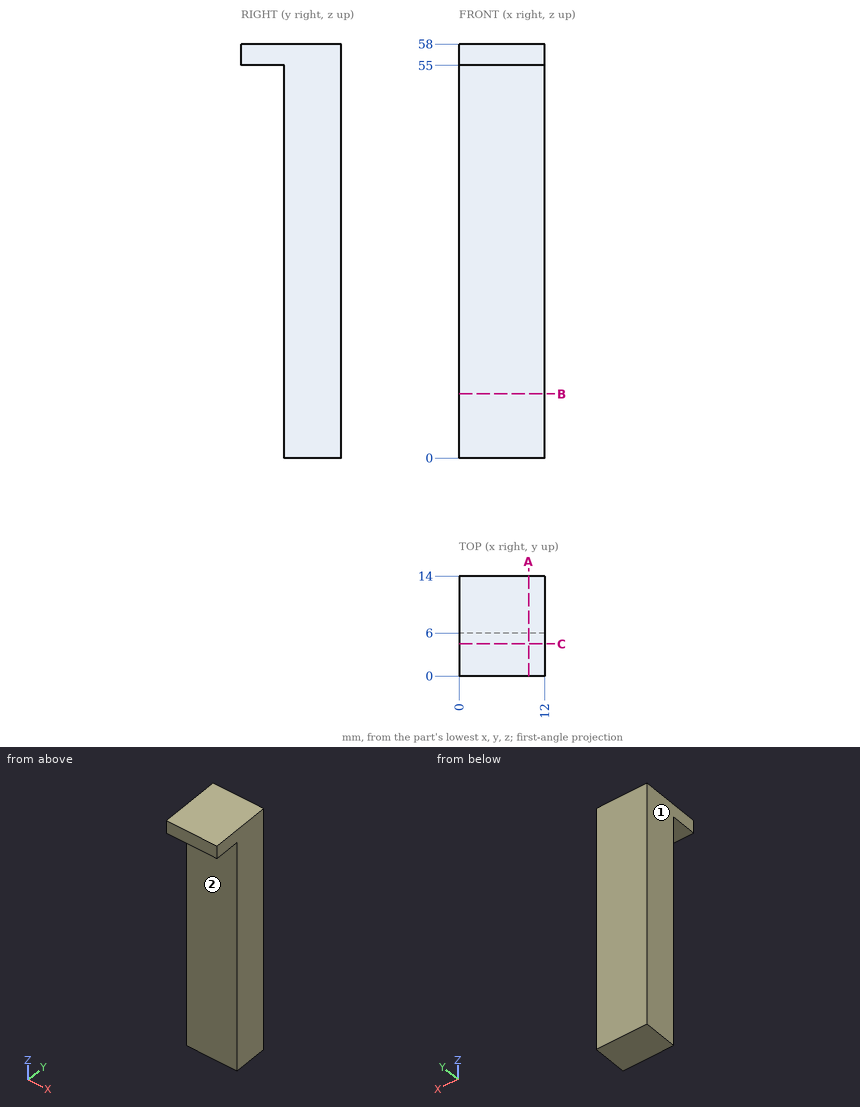
Job drawing, mm, ordinate dimensions from the low corner. One solid piece. A direction names the side the tool comes from. Coordinates: 2 decimals unless noted, no trailing zeros. Order: outer loops, then holes, each group sorted by start corner. A loop starts at its lowest first (then second) coordinate and runs counter-clockwise, first axis right, second up. Notation, with made-up numbers: (14.5, 30) -> (29.5, 30) arc R21 cw to (29.5, 68) -> close; hole circle Ø8 at (0.25, -28.5). An arc over 180 degrees is marked (long way). Return JSON: item names as keys, results as strings. Group by question number.
Item 1: Saw through at C-C on y = 4.5. Write the cut outline in (x, z), then the cut area to 3 significant figures.
Item 2: Flat gauge pins, fed straight in: P1, Ø3, axis at x = 5.5, z = 37, coming from the -Y side; P2, Ø1.8, axis at x = 4, y = 3, coming from the -Z side. Where does each tip first touch, or does it go through?
Item 3: Wall check: line 1 along Y through (x, z) = (10.5, 9); line 2 along Z through (x, y) = (7, 4.5). Give the ranges that are in metal, low to high. Write a range as [from, to].
Item 4: Saw through at A-A on x = 9.75. Write the cut outline in (y, z).
Item 5: Tool access for the marked faces 1 and 2: list every direction of +Z, -Z, +X, -X, +Y, -Y with a clear straight run to the whole face (end or side of a thin tool).
Item 6: Saw through at B-B on z = 9. Write the cut outline in (x, y).
Values found:
{
 "1": {"outline": "(0, 55) -> (12, 55) -> (12, 58) -> (0, 58) -> close", "area": "36.0 mm2"},
 "2": {"P1": "stops at y = 6", "P2": "stops at z = 55"},
 "3": {"line 1": "y = [6, 14]", "line 2": "z = [55, 58]"},
 "4": {"outline": "(0, 55) -> (6, 55) -> (6, 0) -> (14, 0) -> (14, 58) -> (0, 58) -> close"},
 "5": {"face 1": "+Z, -Z, -X, +Y, -Y", "face 2": "-Z, +X, -X, -Y"},
 "6": {"outline": "(0, 6) -> (12, 6) -> (12, 14) -> (0, 14) -> close"}
}
